Could you check a few things on this model? Use its own coordinates, in mm. Face numbers are marked on the shaded views. A direction names the side the tool comes from. Round coordinates to 2 decimals unless told otherwise and drop trailing zeros. Write each loop counter-clockwise with the first axis right and the second up, starting at its lowest first coordinate (ties: lowest second). Pieces come first, ordered by that corner, then holes. Notation, with made-up numbers: M -2.5,84 L 34.5,84 A27 cw 34.5,111 Z; hole C 34.25,69.25 d2. An arc over 180 degrees is marked long. One line per item, written item: value. Start each with the question number.
(1) I want a section at C-C on x = 94. Please give me the cut outline in (y, z).
(2) If I drill on L1, parallel to X at y = -346, z = 255; L2, parallel to Z at x = 45, y = -44.5; L3, parallel to Y at x = -145.5, z = 302, over which ranges is the centre line in solid material (lowest first)?
(3) I'm going to push flat-ended pins straight in: pin 1 Ø1.5 at (x, z) = (-83, 40.5) entering from +Y; pin 2 Ø5 at (y, z) = (-244, -3.5) entering from -X; pin 3 Ø12.5 at (x, y) = (-175, -446.5) entering from +Z. Where does each tip first touch, or does it pass through?
(4) Which directions (+Z, -Z, +X, -X, +Y, -Y) give clear straight access to the entire face, cutting with the end or side of a thin tool? Please do the marked faces 1, 2 and 3.
(5) Thinking about a two-plate mould opening in X: for the marked faces 4, 5, 6 and 7, which applies, released by +X, released by -X, zero draft, split by the parting line, or undercut?
(6) I want a section at D-D on x = -171.5. Please give me the cut outline in (y, z), and give its area (3 significant figures).
(7) I want a section at A-A on y = -78.5. Please give me the cut outline in (x, z), and give its area (3 significant figures).
(8) I want a section at B-B on z = 161.5. Please give me the cut outline in (x, y).
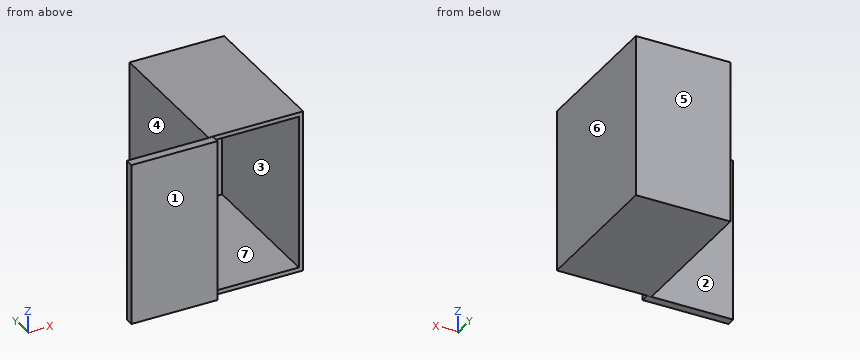
```python
from build123d import *

# Parameters (mm, degrees)
F0_W     = 279.4
F0_H     = 482.6
F1_DEPTH = 431.8
F2_T     = -12.7
F3_W     = 254.188428
F3_H     = 481.781103
F4_DEPTH = 25.4


with BuildPart() as f1:
    # F0 (on Front) → F1 (new body)
    with BuildSketch(Plane.XZ):
        with Locations((121.389246, 165.165817)):
            Rectangle(F0_W, F0_H)
    extrude(amount=F1_DEPTH)

    # F2
    f2_openings = [f1.faces().sort_by_distance(p)[0] for p in [
        (121.389246, -431.8, 165.165817),
    ]]
    offset(amount=F2_T, openings=f2_openings)

    # F3 (on face) → F4 (join)
    with BuildSketch(Plane.XZ.offset(431.8)):
        with Locations((-132.704968, 164.756368)):
            Rectangle(F3_W, F3_H)
    extrude(amount=F4_DEPTH)


solid = f1.part
```
Found:
1. outline: M -431.8,-76.13 L 0,-76.13 L 0,406.47 L -431.8,406.47 L -431.8,393.77 L -12.7,393.77 L -12.7,-63.43 L -431.8,-63.43 Z
2. L1: x = -18.31 to -5.61, 248.39 to 261.09
2. L2: z = -76.13 to -63.43, 393.77 to 406.47
2. L3: y = -457.2 to -431.8
3. pin 1: stops at y = -431.8
3. pin 2: stops at x = -18.31
3. pin 3: stops at z = 405.65
4. face 1: +Z, -Z, +X, -X, -Y
4. face 2: +Z, -Z, -X, +Y
4. face 3: -Y
5. face 4: released by -X
5. face 5: zero draft
5. face 6: released by +X
5. face 7: undercut
6. outline: M -457.2,-76.13 L -431.8,-76.13 L -431.8,405.65 L -457.2,405.65 Z
6. area: 12,200 mm²
7. outline: M -18.31,-76.13 L 261.09,-76.13 L 261.09,406.47 L -18.31,406.47 Z; hole M -5.61,-63.43 L 248.39,-63.43 L 248.39,393.77 L -5.61,393.77 Z
7. area: 18,700 mm²
8. outline: M -259.8,-457.2 L -5.61,-457.2 L -5.61,-12.7 L 248.39,-12.7 L 248.39,-431.8 L 261.09,-431.8 L 261.09,0 L -18.31,0 L -18.31,-431.8 L -259.8,-431.8 Z
